Autodesk Inventor part; units mm, degrees
ref_plane "YZ Plane" through (0, 0, 0) normal (1, 0, 0) x (0, 1, 0)
ref_plane "XZ Plane" through (0, 0, 0) normal (0, 1, 0) x (-1, 0, 0)
ref_plane "XY Plane" through (0, 0, 0) normal (0, 0, 1) x (1, 0, 0)
sketch "Sketch1" plane through (0, 0, 0) normal (0, 0, 1) x (1, 0, 0)
  circle A0 centre (0, 0) radius 260
  circle A1 centre (0, 0) radius 300
  dimension "d0" = 600
  dimension "d1" = 40
extrude "Extrusion1" add sketch "Sketch1" along normal blind 4
sketch "Sketch2" plane through (0, 0, 4) normal (0, 0, 1) x (1, 0, 0)
  line L0 (-300, 0) -> (300, 0)
  line L1 (300, 0) -> (300, -300)
  line L2 (300, -300) -> (-300, -300)
  line L3 (-300, -300) -> (-300, 0)
  circle A0 centre (0, 0) radius 300
  line L4 (-420, 0) -> (420, 0)
extrude "Extrusion2" cut sketch "Sketch2" against normal blind 10 contours L0 A0 picked at (-23.3445, -97.237)
sketch "Sketch3" plane through (0, 0, 4) normal (0, 0, 1) x (1, 0, 0)
  circle A0 centre (-288.2644, 34.2678) radius 1.5
  arc A1 (300, 0) -> (-300, 0) centre (0, 0) ccw
  circle A2 centre (-267.3724, 37.5767) radius 1.5
  line L0 (-420, 0) -> (420, 0)
  circle A3 centre (-284.9918, 52.8272) radius 1.5
  circle A4 centre (-264.0999, 56.1362) radius 1.5
  line L1 (-267.3724, 37.5767) -> (-288.2644, 34.2678)
  line L2 (-288.2644, 34.2678) -> (-284.9918, 52.8272)
  line L3 (-284.9918, 52.8272) -> (-264.0999, 56.1362)
  line L4 (-264.0999, 56.1362) -> (-267.3724, 37.5767)
  line L5 (-264.0999, 56.1362) -> (0, 0)
  line L6 (0, 0) -> (-267.3724, 37.5767)
  dimension "d6" = 3
  dimension "d7" = 3
  dimension "d9" = 270
  dimension "d11" = 3
  dimension "d12" = 3
  dimension "d14" = 270
  dimension "d21" = 109
  dimension "d22" = 20
  dimension "d23" = 8
  dimension "d24" = 12
extrude "Extrusion3" cut sketch "Sketch3" against normal through all contours A0 L2 L1 | L1 L2 A0 | L1 L6 A2 | A2 L4 L1 | L2 L3 A3 | A3 L3 L2 | A2 L6 L4 | L4 L5 A4 | A4 L3 L4 | A4 L5 L3
pattern_circular "Circular Pattern1" count 9 over 160 about axis through (0, 0, 0) along (0, 0, -1) of "Extrusion3"
properties part number "wheel3"
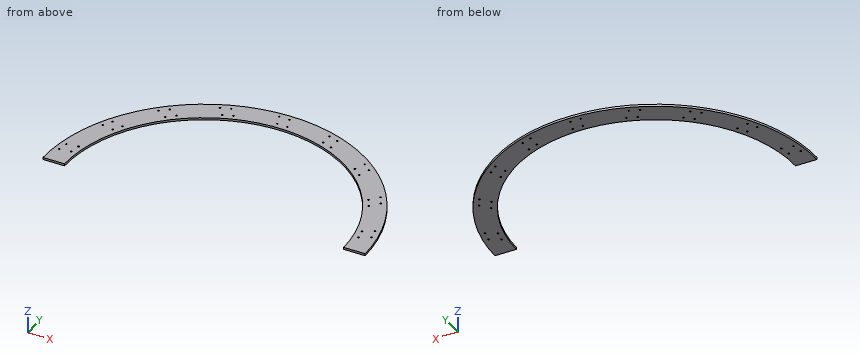
The model under review builds one solid part; all positions refer to its coordinate system, in mm. Coordinates: 2 decimals unless noted, no trailing zeros. Order: outer loops, then holes, each group sorted by start corner. A loop starts at its lowest first (then second) coordinate and runs counter-clockwise, first axis right, second up. Notation, with made-up numbers: (43.25, 25.5) -> (63.25, 25.5) arc R26 ccw to (63.25, 64.5) -> close; hole circle Ø11 at (-28, 73.25). An arc over 180 degrees is marked (long way). Answer in a Markdown table with one row per item. Add a question column.
Item 1: We need section A-A on y = 24. Write out the cut boundary in (x, z).
Item 2: We need section D-D on x = -206. Write out the cut boundary in (y, z).
Item 3: To check wall thickness, follow probe 1 along X at (y, z) = (159.5, 0.95); probe 2 along X at (y, z) = (125.5, 0.6); probe 3 along Y at (x, z) = (-5, 0.3). State the ranges of each line that lie inside material, in increasing order.
Item 4: We need section C-C on y = 176. Write out the cut boundary in (x, z), plus the area to 3 significant figures.
Item 5: Clearance check with flat-ended pins moving along their axes: pin 1 (1.5 mm diameter, centred on y = 120, z = 3, fed in from +X); pin 2 (5 mm diameter, centred on x = -184.36, y = 223.66, fed in from -Z); pin 3 (2 mm diameter, centred on x = -147.5, z = 1, fed in from +Y); pin 4 (1.8 mm diameter, centred on x = 267.37, y = 37.58, fed in from -Z). State where each tip first meets the part, or that it passes through.
Final values:
| question | item | result |
|---|---|---|
| 1 | outline | (-299.04, 0) -> (-258.89, 0) -> (-258.89, 4) -> (-299.04, 4) -> close; (258.89, 0) -> (299.04, 0) -> (299.04, 4) -> (258.89, 4) -> close |
| 2 | outline | (158.63, 0) -> (218.09, 0) -> (218.09, 4) -> (158.63, 4) -> close |
| 3 | probe 1 | x = -254.09 to -205.33, 205.33 to 241.42, 244.28 to 254.09 |
| 3 | probe 2 | x = -272.49 to -239.21, -237.58 to -227.71, 227.71 to 237.58, 239.21 to 272.49 |
| 3 | probe 3 | y = 259.95 to 299.96 |
| 4 | outline | (-242.95, 0) -> (-191.37, 0) -> (-191.37, 4) -> (-242.95, 4) -> close; (191.37, 0) -> (242.95, 0) -> (242.95, 4) -> (191.37, 4) -> close |
| 4 | area | 413 mm2 |
| 5 | pin 1 | stops at x = 275.28 |
| 5 | pin 2 | stops at z = 0 |
| 5 | pin 3 | stops at y = 261.8 |
| 5 | pin 4 | passes through |
